Source: three-view drawing plus pictorial views. Frame: mm from the lowest corner of the part. A direction names the side the tool comes from. Coordinates: 2 decimals unless noted, no trailing zeros. Order: outer loops, then holes, each group sorted by start corner. A loop starts at its lowest first (then second) coordinate and runs counter-clockwise, first axis right, second up. Notation, with made-up numbers: M -15,36 L 29,36 A19 cw 29,67 Z; hole C -32.75,57 d6. An arc over 180 degrees is marked long. One line per question, with ' | ' between items.
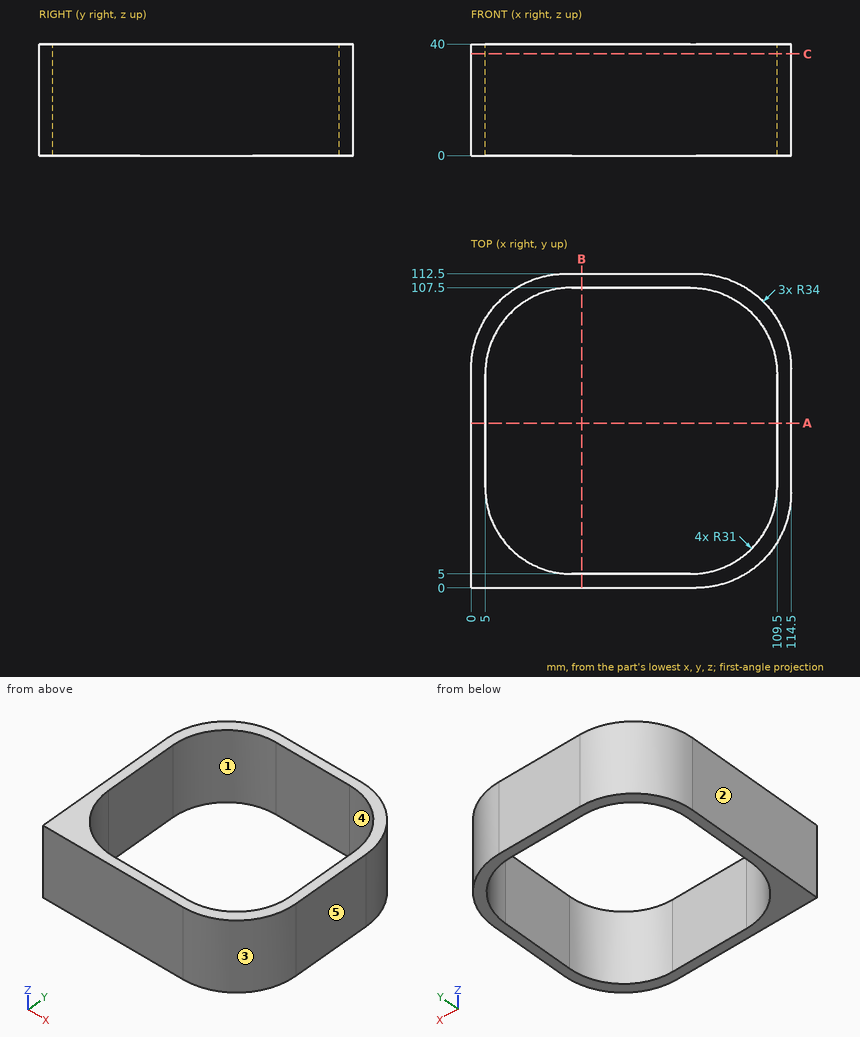
1. Material intervals for line 1 (X direction, y = 40, z = 7); line 2 (Y direction, x = 44, z = 5.5); line 3 (X direction, y = 29, z = 22.5), sorted ascending. Write a range as [from, to].
Response values:
line 1: x = [0, 5], [109.5, 114.5] | line 2: y = [0, 5], [107.5, 112.5] | line 3: x = [0, 5.8], [108.7, 114.13]
2. Section C-C, the plane z = 36.5. Output: boundary loops of the cut face in (x, y).
Response values:
outline: M 0,0 L 80.5,0 A34 ccw 114.5,34 L 114.5,78.5 A34 ccw 80.5,112.5 L 34,112.5 A34 ccw 0,78.5 Z; hole M 5,36 A31 ccw 36,5 L 78.5,5 A31 ccw 109.5,36 L 109.5,76.5 A31 ccw 78.5,107.5 L 36,107.5 A31 ccw 5,76.5 Z
3. Access query for the marked faces 4 and 5. Directions: +Z, -Z, +X, -X, +Y, -Y. A direction counts if a zero-diameter tool reaches every point of the face in a straight line with its end or side. Return the directions, or none.
Response values:
face 4: +Z, -Z | face 5: +Z, -Z, +X, +Y, -Y
4. Section A-A, the plane y = 59. Output: boundary loops of the cut face in (x, z).
Response values:
outline: M 0,0 L 5,0 L 5,40 L 0,40 Z; M 109.5,0 L 114.5,0 L 114.5,40 L 109.5,40 Z
5. Draft query along Y for the marked faces 1, 2 and 3. Return one class per face: pulls with the +Y half, pulls with the -Y half, needs draft (parallel to the pull), parting line crosses it, or undercut.
Response values:
face 1: undercut | face 2: needs draft | face 3: pulls with the -Y half
6. Section B-B, the plane x = 39.5. Output: boundary loops of the cut face in (y, z), and give its area (3 significant figures).
Response values:
outline: M 0,0 L 5,0 L 5,40 L 0,40 Z; M 107.5,0 L 112.5,0 L 112.5,40 L 107.5,40 Z | area: 400 mm^2
